from build123d import *

# Parameters (mm, degrees)
SKETCH1_W                = 13
SKETCH1_H                = 13
BALL_BEARING_BLOCK_DEPTH = 19.5
SKETCH2_W                = 34
SKETCH2_H                = 4
PADDLE_PLATE_DEPTH       = 19.5
SKETCH3_R                = 5.125
BALLBEARING_1_DEPTH      = 4.5
BALLBEARING_START        = -5
SKETCH4_R                = 5.125
BALLBEARING_2_DEPTH      = 5
SKETCH5_R                = 3
ACHSE_DEPTH              = 10
ACHSE_START              = -0.25
SKETCH9_R                = 3
ACHSE_CLOSER_DEPTH       = 0.25
FILLET1_R                = 5
FILLET2_R                = 5
FILLET3_R                = 2
FILLET4_R                = 2
FILLET7_R                = 2
SKETCH6_R                = 1.625
M3_PADDLE_SCREWS_DEPTH   = 4
SKETCH8_W                = 21.5
SKETCH8_H                = 19.5
TOP_PLATE_DEPTH          = 1.5
SKETCH7_R                = 7.75
MAGNET_POCKET_DEPTH      = 3.75


with BuildPart() as part:
    # Sketch1 → Ball Bearing Block (new body)
    with BuildSketch(Plane.XY):
        Rectangle(SKETCH1_W, SKETCH1_H)
    extrude(amount=BALL_BEARING_BLOCK_DEPTH)

    # Sketch2 → Paddle Plate (add)
    with BuildSketch(Plane(origin=(0, 0, 0), x_dir=(1, 0, 0), z_dir=(0, 0, -1))):
        with Locations((-23.5, 0)):
            Rectangle(SKETCH2_W, SKETCH2_H)
    extrude(amount=-PADDLE_PLATE_DEPTH)

    # Sketch3 → Ballbearing 1 (cut)
    with BuildSketch(Plane.XY.offset(19.5)):
        Circle(SKETCH3_R)
    extrude(amount=-BALLBEARING_1_DEPTH, mode=Mode.SUBTRACT)

    # Sketch4 → Ballbearing 2 (cut)
    with BuildSketch(Plane(origin=(0, 0, 0), x_dir=(1, 0, 0), z_dir=(0, 0, -1)).offset(BALLBEARING_START)):
        Circle(SKETCH4_R)
    extrude(amount=BALLBEARING_2_DEPTH, mode=Mode.SUBTRACT)

    # Sketch5 → Achse (cut)
    with BuildSketch(Plane.XY.offset(15)):
        Circle(SKETCH5_R)
    extrude(amount=-ACHSE_DEPTH, mode=Mode.SUBTRACT)

    # Sketch9 → Achse Closer (add)
    with BuildSketch(Plane(origin=(0, 0, 5), x_dir=(-1, 0, 0), z_dir=(0, 0, -1)).offset(ACHSE_START)):
        with Locations(Location((0, 0, 0), (0, 0, 180))):
            Circle(SKETCH9_R)
    extrude(amount=ACHSE_CLOSER_DEPTH)

    # Fillet1
    fillet1_edges = [part.edges().sort_by_distance(p)[0] for p in [
        (6.5, 6.5, 9.75),
    ]]
    fillet(fillet1_edges, radius=FILLET1_R)

    # Fillet2
    fillet2_edges = [part.edges().sort_by_distance(p)[0] for p in [
        (6.5, -6.5, 9.75),
    ]]
    fillet(fillet2_edges, radius=FILLET2_R)

    # Fillet3
    fillet3_edges = [part.edges().sort_by_distance(p)[0] for p in [
        (-6.5, 6.5, 9.75),
    ]]
    fillet(fillet3_edges, radius=FILLET3_R)

    # Fillet4
    fillet4_edges = [part.edges().sort_by_distance(p)[0] for p in [
        (-6.5, -6.5, 9.75),
    ]]
    fillet(fillet4_edges, radius=FILLET4_R)

    # Fillet7
    fillet7_edges = [part.edges().sort_by_distance(p)[0] for p in [
        (-6.5, -2, 9.75),
    ]]
    fillet(fillet7_edges, radius=FILLET7_R)

    # Sketch6 → M3 Paddle Screws (cut)
    with BuildSketch(Plane(origin=(0, 2, 0), x_dir=(-1, 0, 0), z_dir=(0, 1, 0))):
        with Locations(Location((35.5, 4.75, 0), (0, 0, 90))):
            Circle(SKETCH6_R)
        with Locations(Location((35.5, 14.75, 0), (0, 0, 180))):
            Circle(SKETCH6_R)
    extrude(amount=-M3_PADDLE_SCREWS_DEPTH, mode=Mode.SUBTRACT)

    # Sketch8 → Top Plate (add)
    with BuildSketch(Plane(origin=(0, 2, 0), x_dir=(-1, 0, 0), z_dir=(0, 1, 0))):
        with Locations((17.25, 9.75)):
            Rectangle(SKETCH8_W, SKETCH8_H)
    extrude(amount=TOP_PLATE_DEPTH)

    # Sketch7 → Magnet Pocket (cut)
    with BuildSketch(Plane(origin=(0, -2, 0), x_dir=(-1, 0, 0), z_dir=(0, 1, 0))):
        with Locations(Location((19, 9.75, 0), (0, 0, 90))):
            Circle(SKETCH7_R)
    extrude(amount=MAGNET_POCKET_DEPTH, mode=Mode.SUBTRACT)


solid = part.part
Source: CAD feature listing. Evaluate the final solid. Frame: model axes, mm. A direction names the side the tool comes from. Coordinates: 2 decimals unless noted, no trailing zeros. Loops run counter-clockwise (first coordinate to the right, second up) from the corner with the lowest first, then second, coordinate; pieces in that order, holes last. Notation, with made-up numbers: (0, 3.25) -> (8, 3.25) arc R20 ccw to (8, 23.25) -> close; hole circle Ø5 at (40, 40). An arc over 180 degrees is marked (long way). Answer in a Markdown table with one row per item. Add a question column.
Q1. Reachability of faces 1 (the face through (-17, 0, 0)), 2 (the face through (0, 0, 5)), 3 (the face through (-11.316, -0.151, 8.741)), 4 (the face through (-1.111, -5.003, 17.282)) from +Z, -Z, +X, -X, +Y, -Y: full face, straight path, thin tool, end or side. Return the list, or none.
Q2. Section A-A on y = 0. Return the cut outline in (x, z) (3 decimals), and give its area (3 significant figures).
Q3. Section C-C on z = 15.75. Return the cut outline in (x, y) (3 decimals).
Q4. Pull-direction query (Y, two-part tool) for faces 5 (the face through (-34, 2, 10)), 6 (the face through (-6.5, 4, 10)), 7 (the face through (-1.111, 5.003, 2.535)), 8 (the face through (-19, 1.75, 10)); classes: pulls with the +Y half, pulls with the -Y half, needs draft (parallel to the pull), parting line crosses it, or undercut.
Q5. Section B-B on z = 7.25. Return the cut outline in (x, y), and give its area (3 significant figures).
Q6. Ray query, line 1 along X through (y, z) = (0, 1.8) (3 decimals); line 2 along Y through (x, z) = (0, 2.65) (3 decimals); line 3 along X through (y, z) = (0, 3.8) (3 decimals). Return the intervals inside material, ascending.
Q7. Section D-D on x = -25. Return the cut outline in (y, z).
Q8. Contact query for flat-ended pins moving along their axis: pin 1 Ø0.6 at (y, z) = (-4, 14) entering from -X; pin 2 Ø1.5 at (x, z) = (-30, 16.5) entering from -Y; pin 3 Ø3 at (x, y) = (0.5, 1.5) entering from +Z; pin 4 Ø1.9 at (x, z) = (-35.5, 14.75) entering from +Y. Output: stop coordinate, or through.
Computed values:
| question | item | result |
|---|---|---|
| 1 | face 1 | -Z, +X, -X, +Y, -Y |
| 1 | face 2 | -Z |
| 1 | face 3 | -Y |
| 1 | face 4 | +Z |
| 2 | outline | (-40.5, 0) -> (-5.125, 0) -> (-5.125, 5) -> (5.125, 5) -> (5.125, 0) -> (6.5, 0) -> (6.5, 19.5) -> (5.125, 19.5) -> (5.125, 15) -> (3, 15) -> (3, 5.25) -> (-3, 5.25) -> (-3, 15) -> (-5.125, 15) -> (-5.125, 19.5) -> (-40.5, 19.5) -> close; hole circle Ø3.25 at (-35.5, 4.75); hole circle Ø3.25 at (-35.5, 14.75); hole circle Ø15.5 at (-19, 9.75) |
| 2 | area | 555 mm^2 |
| 3 | outline | (-40.5, -2) -> (-36.781, -2) -> (-36.781, 2) -> (-40.5, 2) -> close; (-34.219, -2) -> (-23.905, -2) -> (-23.905, 1.75) -> (-14.095, 1.75) -> (-14.095, -2) -> (-8.5, -2) arc R2 cw to (-6.5, -4) -> (-6.5, -4.5) arc R2 ccw to (-4.5, -6.5) -> (1.5, -6.5) arc R5 ccw to (6.5, -1.5) -> (6.5, 1.5) arc R5 ccw to (1.5, 6.5) -> (-4.5, 6.5) arc R2 ccw to (-6.5, 4.5) -> (-6.5, 3.5) -> (-28, 3.5) -> (-28, 2) -> (-34.219, 2) -> close; hole circle Ø10.25 at (0, 0) |
| 4 | face 5 | pulls with the +Y half |
| 4 | face 6 | needs draft |
| 4 | face 7 | undercut |
| 4 | face 8 | pulls with the -Y half |
| 5 | outline | (-40.5, -2) -> (-26.34, -2) -> (-26.34, 1.75) -> (-11.66, 1.75) -> (-11.66, -2) -> (-8.5, -2) arc R2 cw to (-6.5, -4) -> (-6.5, -4.5) arc R2 ccw to (-4.5, -6.5) -> (1.5, -6.5) arc R5 ccw to (6.5, -1.5) -> (6.5, 1.5) arc R5 ccw to (1.5, 6.5) -> (-4.5, 6.5) arc R2 ccw to (-6.5, 4.5) -> (-6.5, 3.5) -> (-28, 3.5) -> (-28, 2) -> (-40.5, 2) -> close; hole circle Ø6 at (0, 0) |
| 5 | area | 242 mm^2 |
| 6 | line 1 | x = -40.5 to -5.125, 5.125 to 6.5 |
| 6 | line 2 | y = -6.5 to -5.125, 5.125 to 6.5 |
| 6 | line 3 | x = -40.5 to -36.818, -34.182 to -23.966, -14.034 to -5.125, 5.125 to 6.5 |
| 7 | outline | (-2, 0) -> (3.5, 0) -> (3.5, 19.5) -> (-2, 19.5) -> (-2, 14.66) -> (1.75, 14.66) -> (1.75, 4.84) -> (-2, 4.84) -> close |
| 8 | pin 1 | stops at x = -6.52 |
| 8 | pin 2 | stops at y = -2 |
| 8 | pin 3 | stops at z = 15 |
| 8 | pin 4 | passes through |
